Part model, mm, in its own coordinate system. Round coordinates to 2 decimals unless told otherwise and drop trailing zeros. Write each loop counter-clockwise with the first axis right and the second up, starting at its lowest first coordinate (ties: lowest second). Pieces come first, ordered by that corner, then holes.
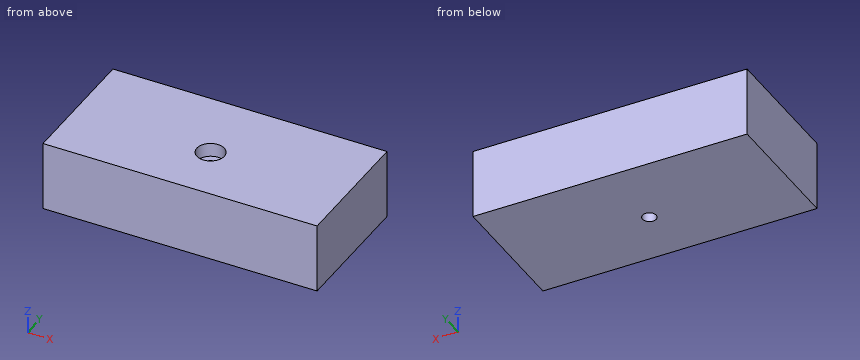
```python
from build123d import *

# Parameters (mm, degrees)
F0_W           = 100
F0_H           = 48
F1_DEPTH       = 25.4
F3_D           = 5
F3_CBORE_D     = 10
F3_CBORE_DEPTH = 5


with BuildPart() as f1:
    # F0 (on Top) → F1 (new body)
    with BuildSketch(Plane.XY):
        with Locations((0, 3.029243)):
            Rectangle(F0_W, F0_H)
    extrude(amount=F1_DEPTH)

    # F3 (through all)
    with Locations(Plane.XY.offset(25.4)):
        with Locations((0, 0)):
            CounterBoreHole(F3_D / 2, F3_CBORE_D / 2, F3_CBORE_DEPTH)


solid = f1.part
```
Q1. Wall check: L1, parallel to Y at x = 0, z = 9.5; L2, parallel to Y at x = 0, z = 22.3; L3, parallel to X at y = 1.5, z = 6.5. Give the ranges that are in metal, low to high.
Values follow:
L1: y = -20.97 to -2.5, 2.5 to 27.03
L2: y = -20.97 to -5, 5 to 27.03
L3: x = -50 to -2, 2 to 50
Q2. Cut at A-A on x = 0. Write the cut outline in (y, z), plus the area to 3 significant figures.
Values follow:
outline: (-20.97, 0) - (-2.5, 0) - (-2.5, 20.4) - (-5, 20.4) - (-5, 25.4) - (-20.97, 25.4) - close; (2.5, 0) - (27.03, 0) - (27.03, 25.4) - (5, 25.4) - (5, 20.4) - (2.5, 20.4) - close
area: 1,070 mm2
Q3. Drop flat-ended pins along their axis: pin 1 (6.5 mm diameter, centred on x = 0, y = 0, fed in from +Z); pin 2 (10 mm diameter, centred on x = -17.5, y = 18.5, fed in from -Z). Give the stop position or say it passes through.
Values follow:
pin 1: stops at z = 20.4
pin 2: stops at z = 0
